```python
from build123d import *

# Parameters (mm, degrees)
ESQUISSE1_W             = 50
ESQUISSE1_H             = 7
BOSS_EXTRU_1_DEPTH      = 28
ESQUISSE2_R             = 1.75
ENL_V_MAT_EXTRU_2_DEPTH = 70
ESQUISSE3_R             = 1.5
ESQUISSE3_W             = 13
ESQUISSE3_H             = 18
ENL_V_MAT_EXTRU_3_DEPTH = 58.732140095


with BuildPart() as part:
    # Esquisse1 → Boss.-Extru.1 (new body)
    with BuildSketch(Plane.XY):
        with Locations((25, 3.5)):
            Rectangle(ESQUISSE1_W, ESQUISSE1_H)
    extrude(amount=BOSS_EXTRU_1_DEPTH)

    # Esquisse2 → Enlèv. mat.-Extru.2 (cut)
    with BuildSketch(Plane.XY.offset(28)):
        with Locations((5.25, 3.5)):
            Circle(ESQUISSE2_R)
        with Locations((44.5, 3.5)):
            Circle(ESQUISSE2_R)
    extrude(amount=-ENL_V_MAT_EXTRU_2_DEPTH, mode=Mode.SUBTRACT)

    # Esquisse3 → Enlèv. mat.-Extru.3 (cut, through all)
    with BuildSketch(Plane(origin=(0, 7, 0), x_dir=(1, 0, 0), z_dir=(0, 1, 0))):
        with Locations(Location((14.5, -6.67085961, 0), (0, 0, 270))):
            Circle(ESQUISSE3_R)
        with Locations(Location((14.5, -18.67085961, 0), (0, 0, 270))):
            Circle(ESQUISSE3_R)
        with Locations(Location((35.5, -6.67085961, 0), (0, 0, 270))):
            Circle(ESQUISSE3_R)
        with Locations(Location((35.5, -18.67085961, 0), (0, 0, 270))):
            Circle(ESQUISSE3_R)
        with Locations((25, -12)):
            Rectangle(ESQUISSE3_W, ESQUISSE3_H)
    extrude(amount=-ENL_V_MAT_EXTRU_3_DEPTH, mode=Mode.SUBTRACT)


solid = part.part
```
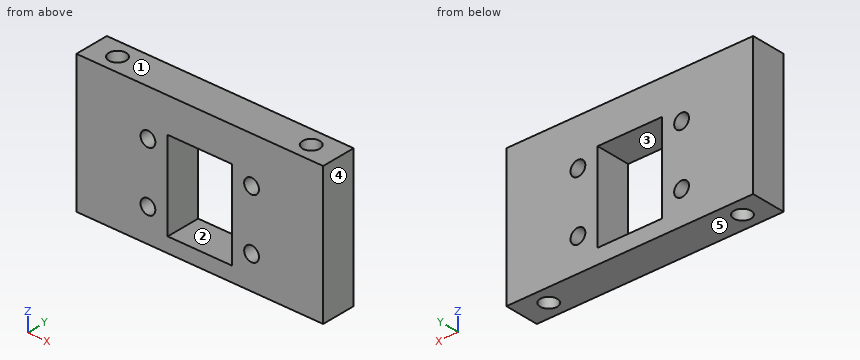
The model under review builds one solid part; all positions refer to its coordinate system, in mm. Face numbers are marked on the shaded views. A direction names the side the tool comes from. Give positions to 0.01 mm unless a question says otherwise; leave off trailing zeros. Order: outer loops, then holes, each group sorted by start corner. A loop starts at its lowest first (then second) coordinate and runs counter-clockwise, first axis right, second up. Notation, with made-up numbers: (-27, 83.5) - (-10, 83.5) arc R24 cw to (-10, 111.5) - close; hole circle Ø2 at (49.5, 26). An arc over 180 degrees is marked (long way). Use CSV: the item, a comma, the result in double quotes. Start each with the question number.
Q1. We need section A-A, the plane x = 5.25. Write out the cut boundary in (y, z), and give its area (3 significant figures).
Q2. Clearance check with a flat-ended pin moving along its axis: pin 1 Ø2 at (y, z) = (5, 9.5) entering from -X. State where the tip first meets the part, or that it passes through.
Q3. To check wall thickness, follow line 1 along Z through (x, y) = (26, 1); line 2 along X through (y, z) = (3.25, 8.25); line 3 along X through (y, z) = (6.25, 12). State the ranges of each line that lie inside material, in increasing order. Write a range as [from, to].
Q4. We need section B-B, the plane y = 3.5. Write out the cut boundary in (x, z), and give its area (3 significant figures).
Q5. We need section C-C, the plane z = 19. Write out the cut boundary in (x, y), and give its area (3 significant figures).
Q6. Tool access review of the marked faces 1 and 2: name each direction out of +Z, -Z, +X, -X, +Y, -Y from which nothing blocks a thin tool from reaching the whole face with its end or side.
Q7. The part is to be moulded in two halves that separate along X. For the marked faces 3, 4 and 5, say which applies: +X half, -X half, draft (parallel to the pull), parting line (faces both ways), or undercut.
Q8. We need section D-D, the plane x = 14.5. Write out the cut boundary in (y, z), and give its area (3 significant figures).
Outcome:
1,outline,"(0, 0) - (1.75, 0) - (1.75, 28) - (0, 28) - close; (5.25, 0) - (7, 0) - (7, 28) - (5.25, 28) - close"
1,area,"98.0 mm^2"
2,pin 1,"stops at x = 0"
3,line 1,"z = [0, 3], [21, 28]"
3,line 2,"x = [0, 3.52], [6.98, 18.5], [31.5, 42.77], [46.23, 50]"
3,line 3,"x = [0, 18.5], [31.5, 50]"
4,outline,"(0, 0) - (3.5, 0) - (3.5, 28) - (0, 28) - close; (7, 0) - (42.75, 0) - (42.75, 28) - (7, 28) - close; (46.25, 0) - (50, 0) - (50, 28) - (46.25, 28) - close; hole circle Ø3 at (14.5, 6.67); hole circle Ø3 at (14.5, 18.67); hole (18.5, 3) - (31.5, 3) - (31.5, 21) - (18.5, 21) - close; hole circle Ø3 at (35.5, 6.67); hole circle Ø3 at (35.5, 18.67)"
4,area,"942 mm^2"
5,outline,"(0, 0) - (13.04, 0) - (13.04, 7) - (0, 7) - close; (15.96, 0) - (18.5, 0) - (18.5, 7) - (15.96, 7) - close; (31.5, 0) - (34.04, 0) - (34.04, 7) - (31.5, 7) - close; (36.96, 0) - (50, 0) - (50, 7) - (36.96, 7) - close; hole circle Ø3.5 at (5.25, 3.5); hole circle Ø3.5 at (44.5, 3.5)"
5,area,"199 mm^2"
6,face 1,"+Z, +X, -X, +Y, -Y"
6,face 2,"+Y, -Y"
7,face 3,"undercut"
7,face 4,"+X half"
7,face 5,"draft"
8,outline,"(0, 0) - (7, 0) - (7, 5.17) - (0, 5.17) - close; (0, 8.17) - (7, 8.17) - (7, 17.17) - (0, 17.17) - close; (0, 20.17) - (7, 20.17) - (7, 28) - (0, 28) - close"
8,area,"154 mm^2"
